Part model, mm, in its own coordinate system. A direction names the side the tool comes from. Give positions to 0.01 mm unless a question says otherwise; leave off trailing zeros. Order: outer loops, then holes, each group sorted by start corner. A loop starts at its lowest first (then second) coordinate and runs counter-clockwise, first axis right, second up. Notation, with made-up numbers: M 81,5 L 85,5 A23 cw 85,21 Z; hole C 24,84.5 d9. An arc over 180 degrees is marked long. Answer as a JSON object with one key per item and string values.
from build123d import *

# Parameters (mm, degrees)
F1_DEPTH   = 50
F2_SIZE2   = 1
F2_SIZE    = 5
F2_2_SIZE2 = 1
F2_2_SIZE  = 5
F3_SIZE2   = 5
F3_SIZE    = 1
F3_2_SIZE2 = 5
F3_2_SIZE  = 1
F4_R       = 1
F7_DEPTH   = 25
F8_DEPTH   = 25


with BuildPart() as f1:
    # F0 (on Top) → F1 (new body, symmetric)
    with BuildSketch(Plane.XY):
        with BuildLine():
            Line((-3, 0), (-22, 0))
            Line((-22, 0), (-22, -1.5))
            Line((-22, -1.5), (-10, -1.5))
            Line((-10, -1.5), (-10, -2.9619401321))
            Line((-10, -2.9619401321), (-8.5, -2.9619401321))
            Line((-8.5, -2.9619401321), (-8.5, -1.5))
            Line((-8.5, -1.5), (-2.5606601718, -1.5))
            Line((-2.5606601718, -1.5), (-7.8245233162, -6.7638631444))
            Line((-7.8245233162, -6.7638631444), (-10, -6.7638631444))
            Line((-10, -6.7638631444), (-10, -8.5))
            Line((-10, -8.5), (-22, -8.5))
            Line((-22, -8.5), (-22, -10))
            Line((-22, -10), (-10, -10))
            Line((-10, -10), (-10, -22))
            Line((-10, -22), (-8.5, -22))
            Line((-8.5, -22), (-8.5, -10))
            Line((-8.5, -10), (-6.7638631444, -10))
            Line((-6.7638631444, -10), (-6.7638631444, -7.8245233162))
            Line((-6.7638631444, -7.8245233162), (-1.5, -2.5606601718))
            Line((-1.5, -2.5606601718), (-1.5, -8.5))
            Line((-1.5, -8.5), (-2.9619401321, -8.5))
            Line((-2.9619401321, -8.5), (-2.9619401321, -10))
            Line((-2.9619401321, -10), (-1.5, -10))
            Line((-1.5, -10), (-1.5, -22))
            Line((-1.5, -22), (0, -22))
            Line((0, -22), (0, -3))
            ThreePointArc((0, -3), (-0.8786796564, -0.8786796564), (-3, 0))
        make_face()
    extrude(amount=F1_DEPTH, both=True)

    # F2
    f2_edges = [f1.edges().sort_by_distance(p)[0] for p in [
        (-22, -10, 0),
    ]]
    f2_side = f1.faces().sort_by_distance((-16, -10, 0))[0]
    chamfer(f2_edges, length=F2_SIZE, length2=F2_SIZE2, reference=f2_side)

    # F2#2
    f2_2_edges = [f1.edges().sort_by_distance(p)[0] for p in [
        (0, -22, 0),
    ]]
    f2_2_side = f1.faces().sort_by_distance((0, -12.5, 0))[0]
    chamfer(f2_2_edges, length=F2_2_SIZE, length2=F2_2_SIZE2, reference=f2_2_side)

    # F3
    f3_edges = [f1.edges().sort_by_distance(p)[0] for p in [
        (-22, 0, 0),
    ]]
    f3_side = f1.faces().sort_by_distance((-22, -0.75, 0))[0]
    chamfer(f3_edges, length=F3_SIZE, length2=F3_SIZE2, reference=f3_side)

    # F3#2
    f3_2_edges = [f1.edges().sort_by_distance(p)[0] for p in [
        (-10, -22, 0),
    ]]
    f3_2_side = f1.faces().sort_by_distance((-9.25, -22, 0))[0]
    chamfer(f3_2_edges, length=F3_2_SIZE, length2=F3_2_SIZE2, reference=f3_2_side)

    # F4
    f4_edges = [f1.edges().sort_by_distance(p)[0] for p in [
        (-2.56066, -1.5, 0),
        (-1.5, -2.56066, 0),
        (-6.763863, -7.824523, 0),
        (-7.824523, -6.763863, 0),
        (-1.5, -8.5, 0),
        (-8.5, -1.5, 0),
    ]]
    fillet(f4_edges, radius=F4_R)

    # F5 (on Front) → F7 (cut)
    with BuildSketch(Plane.XZ):
        Polygon((0, 50), (-22, 50), (-22, 28), align=None)
        Polygon((-22, -28), (-22, -50), (0, -50), align=None)
    extrude(amount=F7_DEPTH, mode=Mode.SUBTRACT)

    # F6 (on Right) → F8 (cut)
    with BuildSketch(Plane.YZ):
        Polygon((-22, 28), (0, 50), (-22, 50), align=None)
        Polygon((-22, -50), (0, -50), (-22, -28), align=None)
    extrude(amount=-F8_DEPTH, mode=Mode.SUBTRACT)


solid = f1.part
1. Cut at B-B on y = -18.25. Give the cut face in (x, z).
Worked answers:
{"outline": "M -9.75,-31.75 L -8.5,-31.75 L -8.5,31.75 L -9.75,31.75 Z; M -1.5,-31.75 L -0.25,-31.75 L -0.25,31.75 L -1.5,31.75 Z"}
2. Pin check, flat tips, straight feed: P1, Ø0.7, axis at x = -2.5, z = 19, coming from the -Y side; P2, Ø8, axis at x = -3.5, y = -12.5, coming from the -Z side; P3, Ø1.3, axis at y = -5.5, z = -4, coming from the -X side; P4, Ø1.5, axis at x = -4, y = -12.5, coming from the -Z side. Stop position of each tip, or through.
Worked answers:
{"P1": "stops at y = -10", "P2": "stops at z = -41.46", "P3": "stops at x = -7.21", "P4": "passes through"}
3. Which spindle directions (+Z, -Z, +X, -X, +Y, -Y) get a long thin tool onto all of the face, cutting with end or side? Do faces 5 (the flat face through (-10, -13, 1)), 6 (the cylindrical face through (-4.045, -2.133, 0.646)), 7 (the flat face through (-10, -8, 1)). Say none if no direction does.
Worked answers:
{"face 5": "+Z, -Z, -X, -Y", "face 6": "+Z, -Z", "face 7": "+Z, -Z, -X"}
4. Cut at A-A on x = -13. Give the cut face in (y, z), plus the area to 3 significant figures.
Worked answers:
{"outline": "M -10,-37 L -8.5,-37 L -8.5,37 L -10,37 Z; M -1.5,-37 L 0,-37 L 0,37 L -1.5,37 Z", "area": "222 mm^2"}
5. Probe line 1 along X through (y, z) = (-11.5, 37); line 2 along X through (y, z) = (-18.5, 18.5). List the from-to ranges inside material, lowest first.
Worked answers:
{"line 1": "x = -10 to -8.5, -1.5 to 0", "line 2": "x = -9.7 to -8.5, -1.5 to -0.3"}
6. Two-plate mould, pull along X, no slides. Class faces 1 (the flat face through (-8.5, -16, 1)), 2 (the flat face through (-9.8, -2.4, -40.2)), 3 (the flat face through (-16, -8.5, 1)), 4 (the flat face through (0, -10, 1)): +X half, -X half, draft (parallel to the pull), parting line (faces both ways), or undercut.
Worked answers:
{"face 1": "undercut", "face 2": "-X half", "face 3": "draft", "face 4": "+X half"}
